from build123d import *

# Parameters (mm, degrees)
F0_W      = 850.9
F0_H      = 25.4
F1_DEPTH  = 5.08
F3_DEPTH  = 5.08
F5_DEPTH  = 5.08
F7_DEPTH  = 5.08
F8_W      = 50.8
F8_H      = 762
F9_DEPTH  = 5.08
F10_R     = 5.08
F11_W     = 76.2
F11_H     = 50.8
F12_DEPTH = 5.08


with BuildPart() as f1:
    # F0 (on Front) → F1 (new body)
    with BuildSketch(Plane.XZ):
        Polygon((50.8, 50.8), (0, 0), (50.8, 0), (50.8, 25.4), align=None)
        Polygon((0, 762), (0, 0), (50.8, 50.8), (50.8, 711.2), align=None)
        Polygon((50.8, 762), (0, 762), (50.8, 711.2), (50.8, 736.6), align=None)
        with Locations((476.25, 12.7)):
            Rectangle(F0_W, F0_H)
        with Locations((476.25, 749.3)):
            Rectangle(F0_W, F0_H)
        Polygon((901.7, 25.4), (901.7, 0), (952.5, 0), (901.7, 50.8), align=None)
        Polygon((952.5, 762), (901.7, 762), (901.7, 736.6), (901.7, 711.2), align=None)
        Polygon((901.7, 50.8), (952.5, 0), (952.5, 762), (901.7, 711.2), align=None)
    extrude(amount=F1_DEPTH)

    # F2 (on face) → F3 (join)
    with BuildSketch(Plane(origin=(0, 0, 0), x_dir=(1, 0, 0), z_dir=(0, 0, -1))):
        Polygon((0, 50.8), (0, 0), (952.5, 0), (952.5, 50.8), (825.5, 50.8), (825.5, 25.4), (127, 25.4), (127, 50.8), align=None)
    extrude(amount=-F3_DEPTH)

    # F4 (on face) → F5 (join)
    with BuildSketch(Plane.XY.offset(762)):
        Polygon((952.5, 0), (0, 0), (0, -50.8), (127, -50.8), (127, -25.4), (825.5, -25.4), (825.5, -50.8), (952.5, -50.8), align=None)
    extrude(amount=-F5_DEPTH)

    # F6 (on face) → F7 (join)
    with BuildSketch(Plane(origin=(0, 0, 0), x_dir=(0, -1, 0), z_dir=(-1, 0, 0))):
        Polygon((0.254638, 756.92), (0.254638, 0), (50.8, 0), (50.8, 762), align=None)
    extrude(amount=-F7_DEPTH)

    # F8 (on face) → F9 (join)
    with BuildSketch(Plane.YZ.offset(952.5)):
        with Locations((-25.4, 381)):
            Rectangle(F8_W, F8_H)
    extrude(amount=-F9_DEPTH)

    # F10
    f10_edges = [f1.edges().sort_by_distance(p)[0] for p in [
        (0, -25.4, 0),
        (5.08, -27.94, 5.08),
        (5.08, -27.94, 756.92),
        (0, -25.4, 762),
        (952.5, -25.4, 762),
        (947.42, -27.94, 756.92),
        (952.5, -25.4, 0),
        (947.42, -27.94, 5.08),
    ]]
    fillet(f10_edges, radius=F10_R)

    # F11 (on face) → F12 (join)
    with BuildSketch(Plane.XZ.offset(5.08)):
        with Locations((863.6, 711.2)):
            Rectangle(F11_W, F11_H)
        with Locations((863.6, 50.8)):
            Rectangle(F11_W, F11_H)
        with Locations((88.9, 50.8)):
            Rectangle(F11_W, F11_H)
        with Locations((88.9, 711.2)):
            Rectangle(F11_W, F11_H)
    extrude(amount=-F12_DEPTH)


solid = f1.part
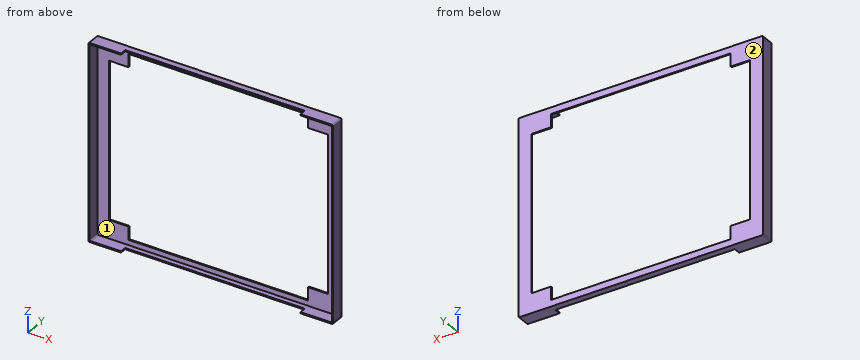
Can you work these out from the model? Positions are in its coordinate system, mm. Face numbers are marked on the shaded views. Give positions to 0.01 mm unless a question says otherwise; leave off trailing zeros. Loops run counter-clockwise (first coordinate to the right, second up) from the corner with the lowest first, then second, coordinate; pieces in that order, holes last. Notation, with made-up numbers: (-34, 56.5) -> (-25, 56.5) arc R7 ccw to (-25, 69.5) -> close; hole circle Ø10 at (33.5, 12). An arc over 180 degrees is marked (long way). Return JSON: item names as keys, results as strings.
Q1. I need wall thicknesses on probe 1 along X at (y, z) = (-38.5, 658.5); probe 2 along Z at (x, y) = (366.5, -9); probe 3 along Z at (x, y) = (436, -3.5). Which ranges of each line are inside material? Lowest first, please.
Checks:
{"probe 1": "x = 0 to 5.08, 947.42 to 952.5", "probe 2": "z = 0 to 5.08, 756.92 to 762", "probe 3": "z = 0 to 25.4, 736.6 to 762"}
Q2. I want a section at A-A, the plane x = 378. List the corners of the cut face in (y, z) for me.
Checks:
{"outline": "(-25.4, 0) -> (0, 0) -> (0, 25.4) -> (-5.08, 25.4) -> (-5.08, 5.08) -> (-25.4, 5.08) -> close; (-25.4, 756.92) -> (-5.08, 756.92) -> (-5.08, 736.6) -> (0, 736.6) -> (0, 762) -> (-25.4, 762) -> close"}
Q3. For pin 1 Ø4 at (y, z) = (-38.5, 2) entering from +X; pin 2 Ø1.5 at (x, z) = (396, 759) entering from -Y; pin 3 Ø1.5 at (y, z) = (-33, 2.5) entering from -X, each with a flat end and sliding along its axis, tell me the tip position at first contact or that it passes through.
Checks:
{"pin 1": "stops at x = 952.38", "pin 2": "stops at y = -25.4", "pin 3": "stops at x = 0.34"}
Q4. I want a section at B-B, the plane y = -36. List the corners of the cut face in (x, z) for me, then the cut area to 3 significant figures.
Checks:
{"outline": "(0, 5.08) arc R5.08 ccw to (5.08, 0) -> (127, 0) -> (127, 5.08) -> (10.16, 5.08) arc R5.08 cw to (5.08, 10.16) -> (5.08, 751.84) arc R5.08 cw to (10.16, 756.92) -> (127, 756.92) -> (127, 762) -> (5.08, 762) arc R5.08 ccw to (0, 756.92) -> close; (825.5, 0) -> (947.42, 0) arc R5.08 ccw to (952.5, 5.08) -> (952.5, 756.92) arc R5.08 ccw to (947.42, 762) -> (825.5, 762) -> (825.5, 756.92) -> (942.34, 756.92) arc R5.08 cw to (947.42, 751.84) -> (947.42, 10.16) arc R5.08 cw to (942.34, 5.08) -> (825.5, 5.08) -> close", "area": "10,200 mm2"}
Q5. I want a section at C-C, the plane z = 186. List the corners of the cut face in (x, y) for me.
Checks:
{"outline": "(0, -50.8) -> (5.08, -50.8) -> (5.08, -5.08) -> (50.8, -5.08) -> (50.8, 0) -> (0, 0) -> close; (901.7, -5.08) -> (947.42, -5.08) -> (947.42, -50.8) -> (952.5, -50.8) -> (952.5, 0) -> (901.7, 0) -> close"}
Q6. We'd pull the mould along X, two halves only. Please class the marked faces 1 and 2: released by +X, released by -X, zero draft, split by the parting line, or undercut.
Checks:
{"face 1": "undercut", "face 2": "zero draft"}
